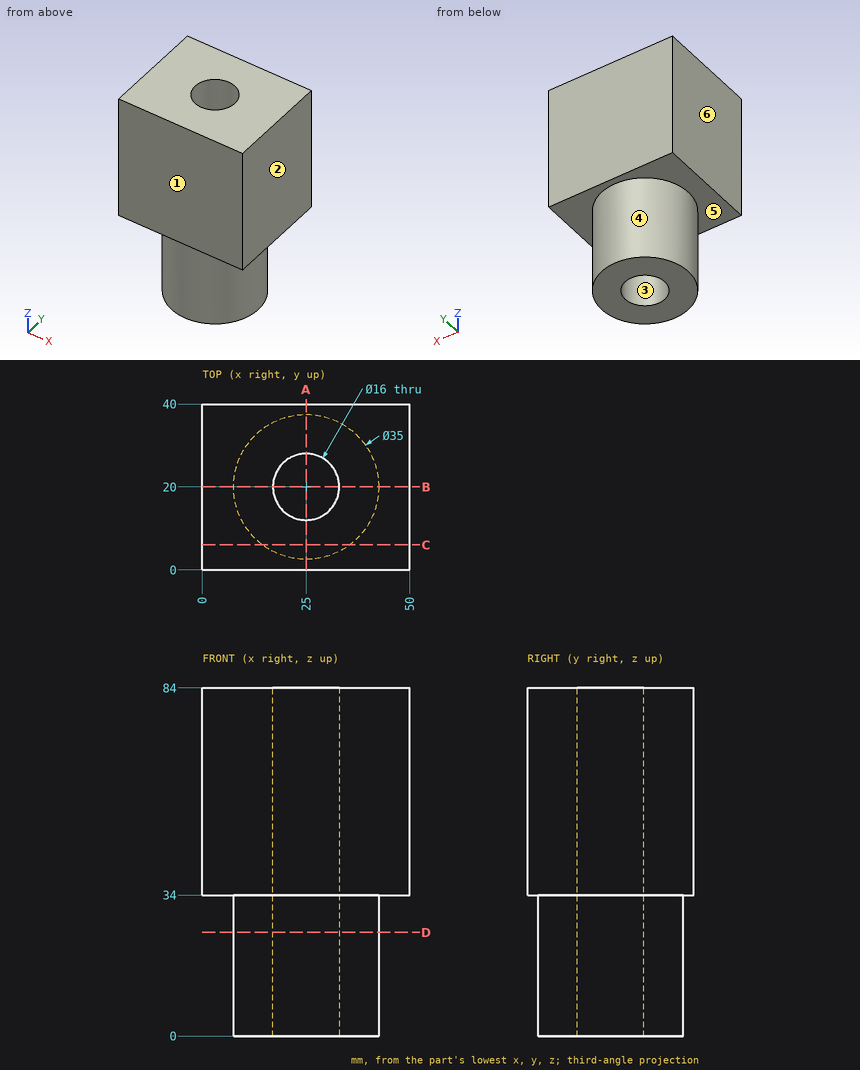
The drawing under review shows one solid part. Ordinate dimensions are in mm from its lowest x, y, z. A direction names the side the tool comes from. Give positions to 0.01 mm unless a question says otherwise; leave off trailing zeros. Loops run counter-clockwise (first coordinate to the right, second up) from the corner with the lowest first, then second, coordinate; pieces in that order, holes last. Notation, with made-up numbers: M -24,9.5 L 16,9.5 A20 cw 16,47.5 Z; hole C -6,-28 d6. An arc over 180 degrees is marked long. Return JSON: item names as keys, results as strings. Group by question number.
Item 1: Mouldability with a two-part tool opening along X and no side actions: class the marked faces 1, 2, 3 and 4 as released by +X, released by -X, zero draft, split by the parting line, or undercut.
Item 2: We need section A-A (x = 25). Give the boundary of the cut face in (y, z).
Item 3: We need section B-B (y = 20). Give the boundary of the cut face in (x, z), and give its area (3 significant figures).
Item 4: Insertion check: pin 1 Ø1 at (x, z) = (25.5, 17.5) entering from -Y; pin 2 Ø1.5 at (y, z) = (7.5, 18.5) entering from -X; pin 3 Ø8 at (x, z) = (30.5, 8.5) entering from +Y. Each pin has a flat end and moves straight along its axis. Give the tip position at first contact, or say it passes through.
Item 5: We need section D-D (z = 25). Give the boundary of the cut face in (x, y), and give its area (3 significant figures).
Item 6: We need section C-C (y = 6). Give the boundary of the cut face in (x, z).
Item 7: Tool access review of the marked faces 5 and 6: name each direction out of +Z, -Z, +X, -X, +Y, -Y from which nothing blocks a thin tool from reaching the whole face with its end or side.
Item 8: For probe 1 along Y at (x, z) = (25, 45); probe 2 along Y at (x, z) = (25, 25); probe 3 along X at (y, z) = (22, 15), list the stretches that pass through material, from the lowest coordinate up.
Output:
{
 "1": {"face 1": "zero draft", "face 2": "released by +X", "face 3": "undercut", "face 4": "split by the parting line"},
 "2": {"outline": "M 0,34 L 2.5,34 L 2.5,0 L 12,0 L 12,84 L 0,84 Z; M 28,0 L 37.5,0 L 37.5,34 L 40,34 L 40,84 L 28,84 Z"},
 "3": {"outline": "M 0,34 L 7.5,34 L 7.5,0 L 17,0 L 17,84 L 0,84 Z; M 33,0 L 42.5,0 L 42.5,34 L 50,34 L 50,84 L 33,84 Z", "area": "2,350 mm^2"},
 "4": {"pin 1": "stops at y = 2.5", "pin 2": "stops at x = 12.03", "pin 3": "stops at y = 37.44"},
 "5": {"outline": "C 25,20 d35; hole C 25,20 d16", "area": "761 mm^2"},
 "6": {"outline": "M 0,34 L 14.5,34 L 14.5,0 L 35.5,0 L 35.5,34 L 50,34 L 50,84 L 0,84 Z"},
 "7": {"face 5": "-Z", "face 6": "+Z, -Z, -X, +Y, -Y"},
 "8": {"probe 1": "y = 0 to 12, 28 to 40", "probe 2": "y = 2.5 to 12, 28 to 37.5", "probe 3": "x = 7.61 to 17.25, 32.75 to 42.39"}
}
